from build123d import *

# Parameters (mm, degrees)
SKETCH_1_W          = 25
SKETCH_1_H          = 60
SKETCH_1_R          = 4.75
SKETCH_1_R_2        = 7.5
EXTRUDE_1_DEPTH     = 48
SKETCH_2_R          = 1.5
CUT_EXTRUDE_1_DEPTH = 10
CUT_EXTRUDE_START   = -10
SKETCH_3_R          = 1.5
CUT_EXTRUDE_2_DEPTH = 10
CHAMFER_1_SIZE      = 5
SKETCH_4_R          = 2.5
CUT_EXTRUDE_3_DEPTH = 5
SKETCH_5_R          = 1.5
CUT_EXTRUDE_4_DEPTH = 5


with BuildPart() as part:
    # 草图1 → 凸台-拉伸1 (new body)
    with BuildSketch(Plane(origin=(0, 0, 0), x_dir=(0, 0, -1), z_dir=(1, 0, 0))):
        Rectangle(SKETCH_1_W, SKETCH_1_H)
        Circle(SKETCH_1_R, mode=Mode.SUBTRACT)
        with Locations((0, 21.5)):
            Circle(SKETCH_1_R_2, mode=Mode.SUBTRACT)
        with Locations((0, -21.5)):
            Circle(SKETCH_1_R_2, mode=Mode.SUBTRACT)
    extrude(amount=EXTRUDE_1_DEPTH)

    # 草图2 → 切除-拉伸1 (cut)
    with BuildSketch(Plane.ZY):
        with Locations((8, 0)):
            Circle(SKETCH_2_R)
        with Locations((-8, 0)):
            Circle(SKETCH_2_R)
    extrude(amount=-CUT_EXTRUDE_1_DEPTH, mode=Mode.SUBTRACT)

    # 草图3 → 切除-拉伸2 (cut)
    with BuildSketch(Plane(origin=(48, 0, 0), x_dir=(0, 0, -1), z_dir=(1, 0, 0)).offset(CUT_EXTRUDE_START)):
        with Locations(Location((8, 0, 0), (0, 0, 180))):
            Circle(SKETCH_3_R)
        with Locations(Location((-8, 0, 0), (0, 0, 180))):
            Circle(SKETCH_3_R)
    extrude(amount=CUT_EXTRUDE_2_DEPTH, mode=Mode.SUBTRACT)

    # 倒角1
    chamfer_1_edges = [part.edges().sort_by_distance(p)[0] for p in [
        (24, 30, 12.5),
        (24, 30, -12.5),
        (24, -30, -12.5),
        (24, -30, 12.5),
    ]]
    chamfer(chamfer_1_edges, length=CHAMFER_1_SIZE)

    # 草图4 → 切除-拉伸3 (cut)
    with BuildSketch(Plane.XY.offset(12.5)):
        with Locations((5, 10)):
            Circle(SKETCH_4_R)
        with Locations(Location((43, 10, 0), (0, 0, 180))):
            Circle(SKETCH_4_R)
    extrude(amount=-CUT_EXTRUDE_3_DEPTH, mode=Mode.SUBTRACT)

    # 草图5 → 切除-拉伸4 (cut)
    with BuildSketch(Plane(origin=(0, 0, -12.5), x_dir=(-1, 0, 0), z_dir=(0, 0, -1))):
        with Locations(Location((-10, 9.5, 0), (0, 0, 90))):
            Circle(SKETCH_5_R)
        with Locations(Location((-10, -9.5, 0), (0, 0, 270))):
            Circle(SKETCH_5_R)
    extrude(amount=-CUT_EXTRUDE_4_DEPTH, mode=Mode.SUBTRACT)


solid = part.part
Work out the finished part from the listing and answer in its coordinate system (mm). A direction names the side the tool comes from. Round coordinates to 2 decimals unless told otherwise and drop trailing zeros. Write each loop counter-clockwise with the first axis right and the second up, starting at its lowest first coordinate (ties: lowest second). Pieces come first, ordered by that corner, then holes. Notation, with made-up numbers: (-20.5, 57.25) -> (19.5, 57.25) arc R9 ccw to (19.5, 74.25) -> close; hole circle Ø1 at (82, 47.25). An arc over 180 degrees is marked (long way). Write each question's results on one line, items separated by ' | '.
Item 1: A cutting plane is placed at C-C, the plane x = 21. Determine the outline of the cut face in (y, z).
Result set:
outline: (-30, -7.5) -> (-25, -12.5) -> (25, -12.5) -> (30, -7.5) -> (30, 7.5) -> (25, 12.5) -> (-25, 12.5) -> (-30, 7.5) -> close; hole circle Ø15 at (-21.5, 0); hole circle Ø9.5 at (0, 0); hole circle Ø15 at (21.5, 0)
Item 2: Which of the six approach directions +Z, -Z, +X, -X, +Y, -Y give full straight-line access (tool end or side, diameter ignored) to faces 1 (the face through (4.93, 0.07, 6.5)), 2 (the face through (43, 10, 7.5)), 3 (the face through (42.93, -0.07, 6.5)), 4 (the face through (23.7, -27.5, 10)), 5 (the face through (10, 9, -7.5))?
Result set:
face 1: -X | face 2: +Z | face 3: +X | face 4: +Z, +X, -X, -Y | face 5: -Z
Item 3: A cutting plane is placed at A-A, the plane y = 21.5. Determine the outline of the cut face in (x, z).
Result set:
outline: (0, -12.5) -> (48, -12.5) -> (48, -7.5) -> (0, -7.5) -> close; (0, 7.5) -> (48, 7.5) -> (48, 12.5) -> (0, 12.5) -> close
Item 4: A cutting plane is placed at B-B, the plane z = 0. Determine the outline of the cut face in (x, y), plus the area to 3 significant figures.
Result set:
outline: (0, -30) -> (48, -30) -> (48, -29) -> (0, -29) -> close; (0, -14) -> (48, -14) -> (48, -4.75) -> (0, -4.75) -> close; (0, 4.75) -> (48, 4.75) -> (48, 14) -> (0, 14) -> close; (0, 29) -> (48, 29) -> (48, 30) -> (0, 30) -> close | area: 984 mm^2
Item 5: Flat-ended cylindrical pins translate along their axes: P1, Ø1.5, axis at y = 0.5, z = -8, coming from the +X side; P2, Ø0.9, axis at y = 0, z = -8.5, coming from the -X side; P3, Ø0.9, axis at x = 10, y = 9.5, coming from the -Z side. Find the tip coordinate at first contact, or state that the pin passes through.
Result set:
P1: x = 38 | P2: x = 10 | P3: z = -7.5
Item 6: Find the intervals of material crossed by line 1 along Y through (x, z) = (21.5, -3.75); line 2 along Y through (x, z) = (34, 0.5); line 3 along Y through (x, z) = (5.5, 8), in increasing order. Write a range as [from, to].
Result set:
line 1: [-30, -28], [-15, -2.92], [2.92, 15], [28, 30] | line 2: [-30, -28.98], [-14.02, -4.72], [4.72, 14.02], [28.98, 30] | line 3: [-29.5, -1.5], [1.5, 7.55], [12.45, 29.5]
Item 7: The mould has two halves that part along X. Classify faces 6 (the face through (38, 0, 8)), 7 (the face through (10, 0, 8)), 8 (the face through (40.69, 10.96, 10.04)), 9 (the face through (24, 0, 12.5)): +X half, -X half, draft (parallel to the pull), parting line (faces both ways), or undercut.
Result set:
face 6: +X half | face 7: -X half | face 8: undercut | face 9: draft
Item 8: A cutting plane is placed at D-D, the plane x = 43. Determine the outline of the cut face in (y, z), plus the area to 3 significant figures.
Result set:
outline: (-30, -7.5) -> (-25, -12.5) -> (25, -12.5) -> (30, -7.5) -> (30, 7.5) -> (25, 12.5) -> (12.5, 12.5) -> (12.5, 7.5) -> (7.5, 7.5) -> (7.5, 12.5) -> (-25, 12.5) -> (-30, 7.5) -> close; hole circle Ø15 at (-21.5, 0); hole circle Ø9.5 at (0, 0); hole circle Ø3 at (0, -8); hole circle Ø3 at (0, 8); hole circle Ø15 at (21.5, 0) | area: 987 mm^2
